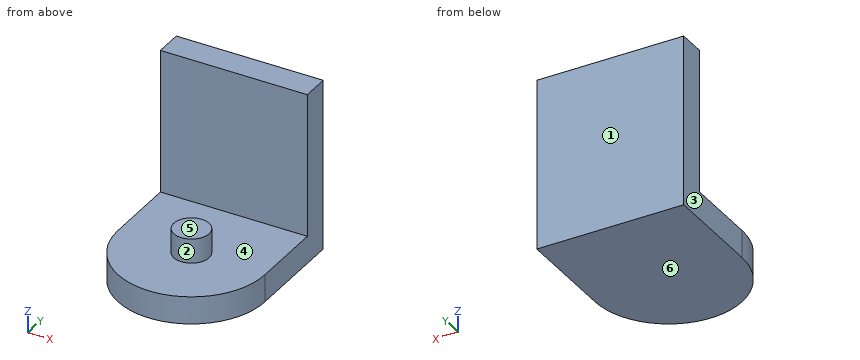
from build123d import *

# Parameters (mm, degrees)
F1_DEPTH = 9.525
F0_W     = 50.8
F0_H     = 9.525
F2_DEPTH = 59.2582
F3_R     = 6.096
F4_DEPTH = 8.4582


with BuildPart() as f1:
    # F0 (on Top) → F1 (new body)
    with BuildSketch(Plane.XY):
        with BuildLine():
            Line((25.4, 25.4), (-25.4, 25.4))
            Line((-25.4, 25.4), (-25.4, 0))
            ThreePointArc((-25.4, 0), (0, -25.4), (25.4, 0))
            Line((25.4, 0), (25.4, 25.4))
        make_face()
    extrude(amount=F1_DEPTH)

    # F0 (on Top) → F2 (join)
    with BuildSketch(Plane.XY):
        with Locations((0, 30.1625)):
            Rectangle(F0_W, F0_H)
    extrude(amount=F2_DEPTH)

    # F3 (on face) → F4 (join)
    with BuildSketch(Plane.XY.offset(9.525)):
        Circle(F3_R)
    extrude(amount=F4_DEPTH)


solid = f1.part
Here's how the part is built. I have some questions about the finished solid (model axes, mm). Face numbers are marked on the shaded views. A direction names the side the tool comes from. Coordinates: 2 decimals unless noted, no trailing zeros. Loops run counter-clockwise (first coordinate to the right, second up) from the corner with the lowest first, then second, coordinate; pieces in that order, holes last. Notation, with made-up numbers: (65, 43.25) -> (81, 43.25) arc R9 cw to (81, 60.25) -> close; hole circle Ø2 at (87.25, 58). An arc over 180 degrees is marked (long way). Use one line per item in the form item = value. Start each with the question number.
(1) If we section it at D-D (y = 2): Please give me the cut outline in (x, z) (3 decimals).
(2) Please list where these lines run through material, in increasing order: line 1 along Z through (x, y) = (-7.5, 12.5) (3 decimals); line 2 along Y through (x, z) = (4.5, 48) (3 decimals); line 3 along Z through (x, y) = (1, -5).
(3) If we section it at B-B (z = 16.5): Please give me the cut outline in (x, y) (3 decimals).
(4) If we section it at C-C (z = 8): Please give me the cut outline in (x, y) (3 decimals), then the cut area to 3 significant figures.
(5) On a 3-axis mill with a long thin cutter (end or side, diameter ignored), from which of +Z, -Z, +X, -X, +Y, -Y can I reach the whole of each face in a straight line? I mean the marked faces 4, 5 and 6. Say none if no direction works.
(6) We'd pull the mould along Y, two halves only. Please class the marked faces 1, 2 and 3: pulls with the +Y half, pulls with the -Y half, needs draft (parallel to the pull), parting line crosses it, or undercut.
(7) Will these pins go through, and if not, where does the flat tip stop? pin 1 (13.5 mm diameter, centred on x = 1, y = -0.5, fed in from +Z); pin 2 (12 mm diameter, centred on x = 14.5, y = 15.5, fed in from +Z) (3 decimals); pin 3 (3 mm diameter, centred on x = -19, z = 31, fed in from -Y).
(8) If we section it at A-A (x = 0): Please give me the cut outline in (y, z) (3 decimals).
Verdict:
q1.outline = (-25.4, 0) -> (25.4, 0) -> (25.4, 9.525) -> (5.759, 9.525) -> (5.759, 17.983) -> (-5.759, 17.983) -> (-5.759, 9.525) -> (-25.4, 9.525) -> close
q2.line_1 = 0 to 9.525
q2.line_2 = 25.4 to 34.925
q2.line_3 = 0 to 17.98
q3.outline = (-25.4, 25.4) -> (25.4, 25.4) -> (25.4, 34.925) -> (-25.4, 34.925) -> close; circle Ø12.192 at (0, 0)
q4.outline = (-25.4, 0) arc R25.4 ccw to (25.4, 0) -> (25.4, 34.925) -> (-25.4, 34.925) -> close
q4.area = 2,790 mm²
q5.face_4 = +Z
q5.face_5 = +Z, +X, -X, -Y
q5.face_6 = -Z, +X, -X, +Y, -Y
q6.face_1 = pulls with the +Y half
q6.face_2 = undercut
q6.face_3 = needs draft
q7.pin_1 = 17.98
q7.pin_2 = 9.525
q7.pin_3 = 25.4
q8.outline = (-25.4, 0) -> (34.925, 0) -> (34.925, 59.258) -> (25.4, 59.258) -> (25.4, 9.525) -> (6.096, 9.525) -> (6.096, 17.983) -> (-6.096, 17.983) -> (-6.096, 9.525) -> (-25.4, 9.525) -> close
